from build123d import *

# Parameters (mm, degrees)
SKETCH1_W           = 146
SKETCH1_H           = 50
BOSS_EXTRUDE1_DEPTH = 5
BOSS_EXTRUDE2_DEPTH = 146
SKETCH4_R           = 3.175
CUT_EXTRUDE1_DEPTH  = 25
SKETCH11_R          = 2
CUT_EXTRUDE3_DEPTH  = 10
SKETCH13_W          = 106
SKETCH13_H          = 65
CUT_EXTRUDE5_DEPTH  = 35
FILLET1_R           = 0.5
FILLET2_R           = 1


with BuildPart() as part:
    # Sketch1 → Boss-Extrude1 (new body)
    with BuildSketch(Plane(origin=(0, 0, 0), x_dir=(1, 0, 0), z_dir=(0, 1, 0))):
        with Locations((73, 25)):
            Rectangle(SKETCH1_W, SKETCH1_H)
    extrude(amount=BOSS_EXTRUDE1_DEPTH)

    # Sketch10 → Boss-Extrude2 (add)
    with BuildSketch(Plane(origin=(146, 0, 0), x_dir=(0, 0, -1), z_dir=(1, 0, 0))):
        Polygon((-25, 0), (-25, -40), (-15, -40), (50, -10), (50, 0), align=None)
        Polygon((-15, -34.493146), (-15, -5), (40, -5), (40, -9.10853), align=None, mode=Mode.SUBTRACT)
    extrude(amount=-BOSS_EXTRUDE2_DEPTH)

    # Sketch4 → Cut-Extrude1 (cut)
    with BuildSketch(Plane(origin=(0, 5, 0), x_dir=(1, 0, 0), z_dir=(0, 1, 0))):
        with Locations((9.5, 37.7)):
            Circle(SKETCH4_R)
        with Locations((9.5, 12.3)):
            Circle(SKETCH4_R)
        with Locations((136.5, 12.3)):
            Circle(SKETCH4_R)
        with Locations((136.5, 37.7)):
            Circle(SKETCH4_R)
    extrude(amount=-CUT_EXTRUDE1_DEPTH, mode=Mode.SUBTRACT)

    # Sketch11 → Cut-Extrude3 (cut)
    with BuildSketch(Plane.XY.offset(25)):
        with Locations((121, -30)):
            Circle(SKETCH11_R)
        with Locations((65, -30)):
            Circle(SKETCH11_R)
        with Locations((65, -10)):
            Circle(SKETCH11_R)
        with Locations((121, -10)):
            Circle(SKETCH11_R)
    extrude(amount=-CUT_EXTRUDE3_DEPTH, mode=Mode.SUBTRACT)

    # Sketch13 → Cut-Extrude5 (cut)
    with BuildSketch(Plane.XZ.offset(40)):
        with Locations((73, -17.5)):
            Rectangle(SKETCH13_W, SKETCH13_H)
    extrude(amount=-CUT_EXTRUDE5_DEPTH, mode=Mode.SUBTRACT)

    # Fillet1
    fillet1_edges = [part.edges().sort_by_distance(p)[0] for p in [
        (73, -5, 15),
        (10, -34.493146, 15),
        (136, -34.493146, 15),
        (15.844375, -9.10853, -40),
        (15.844375, -5, -40),
        (130.155625, -9.10853, -40),
        (130.155625, -5, -40),
        (142.344375, -5, -40),
        (142.344375, -9.10853, -40),
        (3.655625, -5, -40),
        (3.655625, -9.10853, -40),
    ]]
    fillet(fillet1_edges, radius=FILLET1_R)

    # Fillet2
    fillet2_edges = [part.edges().sort_by_distance(p)[0] for p in [
        (73, 0, 25),
        (73, 5, -50),
        (10, -10, -50),
        (73, -40, 25),
        (73, 5, 0),
        (136, -10, -50),
    ]]
    fillet(fillet2_edges, radius=FILLET2_R)


solid = part.part
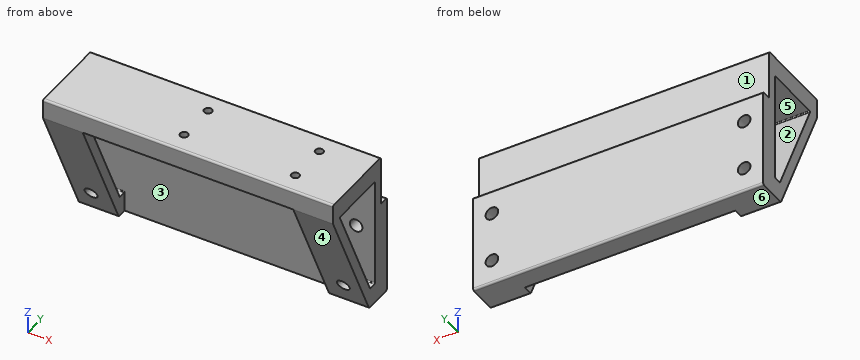
For this review, take the finished solid that the model builds, in its own axes (mm). Face numbers are marked on the shaded views. A direction names the side the tool comes from. Give positions to 0.01 mm unless a question says otherwise; leave off trailing zeros. Loops run counter-clockwise (first coordinate to the right, second up) from the corner with the lowest first, then second, coordinate; pieces in that order, holes last. Notation, with made-up numbers: M -36,88 L -32,88 A20 cw -32,122 Z; hole C -35.5,6.25 d5. An arc over 180 degrees is marked long. Put each result on its own line as item: value. Start each with the question number.
(1) Add section D-D, the plane z = -12.3. Write out the cut boundary in (x, y) (3 decimals).
(2) Add section A-A, the plane x = 57.5. Write out the cut boundary in (y, z).
(3) Add section C-C, the plane y = -30. Write out the cut boundary in (x, z).
(4) Machinability: for the marked faces 5 and 6, which of the approach directions +Z, -Z, +X, -X, +Y, -Y give a long, thin tool a straight path to every point of the face, cutting with its end or side? Answer none if there is none.
(5) For pin 1 (7.5 mm diameter, centred on x = 136.5, z = -37.7, fed in from +Y); pin 2 (5 mm diameter, centred on x = 121, y = -10, fed in from -Z); pin 3 (3 mm diameter, centred on x = 59.5, z = -2, fed in from -Y); pin 4 (2 mm diameter, centred on y = -24, z = -2.5, fed in from +X), all flat-tipped, find the tip position at first contact; note any pin that passes through.
(6) The part is to be moulded in two halves that separate along Y. For the marked faces 1, 2, 3 and 4, say which applies: +Y half, -Y half, draft (parallel to the pull), parting line (faces both ways), or undercut.
(7) Add section B-B, the plane z = -28. Write out the cut boundary in (x, y).
(8) Wall thickness on L1, parallel to X at y = -0.75, z = -12.3 (3 decimals); L2, parallel to Y at x = 121, z = 19.25; L3, parallel to Z at x = 136.5, y = -1.5 (3 decimals): over which ranges is each line inside the solid? List them lowest first.
Result:
1. outline: M 0,-27.4 L 20,-27.4 L 20,-21.893 L 0,-21.893 Z; M 0,-5 L 6.325,-5 L 6.325,5 L 0,5 Z; M 12.675,-5 L 133.325,-5 L 133.325,5 L 12.675,5 Z; M 126,-27.4 L 146,-27.4 L 146,-21.893 L 126,-21.893 Z; M 139.675,-5 L 146,-5 L 146,5 L 139.675,5 Z
2. outline: M -40,15 L -5.5,15 A0.5 cw -5,14.5 L -5,-50 L 4,-50 A1 ccw 5,-49 L 5,-1 A1 ccw 4,0 L 0,0 L 0,24 A1 ccw -1,25 L -39,25 A1 ccw -40,24 Z
3. outline: M 0,-6.67 L 20,-6.67 L 20,5.26 L 0,5.26 Z; M 0,15 L 63,15 L 63,25 L 0,25 Z; M 67,15 L 119,15 L 119,25 L 67,25 Z; M 123,15 L 146,15 L 146,25 L 123,25 Z; M 126,-6.67 L 146,-6.67 L 146,5.26 L 126,5.26 Z
4. face 5: none
4. face 6: -Z, +X, -X, +Y, -Y
5. pin 1: stops at y = 5
5. pin 2: stops at z = 15
5. pin 3: stops at y = -5
5. pin 4: passes through
6. face 1: +Y half
6. face 2: undercut
6. face 3: undercut
6. face 4: -Y half
7. outline: M 0,-20.15 L 20,-20.15 L 20,-14.65 L 0,-14.65 Z; M 0,-5 L 146,-5 L 146,5 L 0,5 Z; M 126,-20.15 L 146,-20.15 L 146,-14.65 L 126,-14.65 Z
8. L1: x = 0 to 6.325, 12.675 to 133.325, 139.675 to 146
8. L2: y = -40 to -32, -28 to -12, -8 to 0
8. L3: z = -50 to -40.875, -34.525 to -15.475, -9.125 to 25
